Geometry: see drawing. Coordinates: mm, zero at the bounding-box minimum. A direction names the side the tool comes from. Give positions to 0.01 mm unless a question says otherwise; leave off trailing zeros. Loops run counter-clockwise (first coordinate to the right, second up) from the corner with the lowest first, then second, coordinate; pieces in that order, holes last. Notation, with made-up numbers: (89, 70.25) -> (132, 70.25) arc R31 cw to (132, 95.25) -> close; hole circle Ø10 at (-31.5, -4). An arc over 180 degrees is marked (long way). Answer in a Markdown table with one row per item. Add a question column.
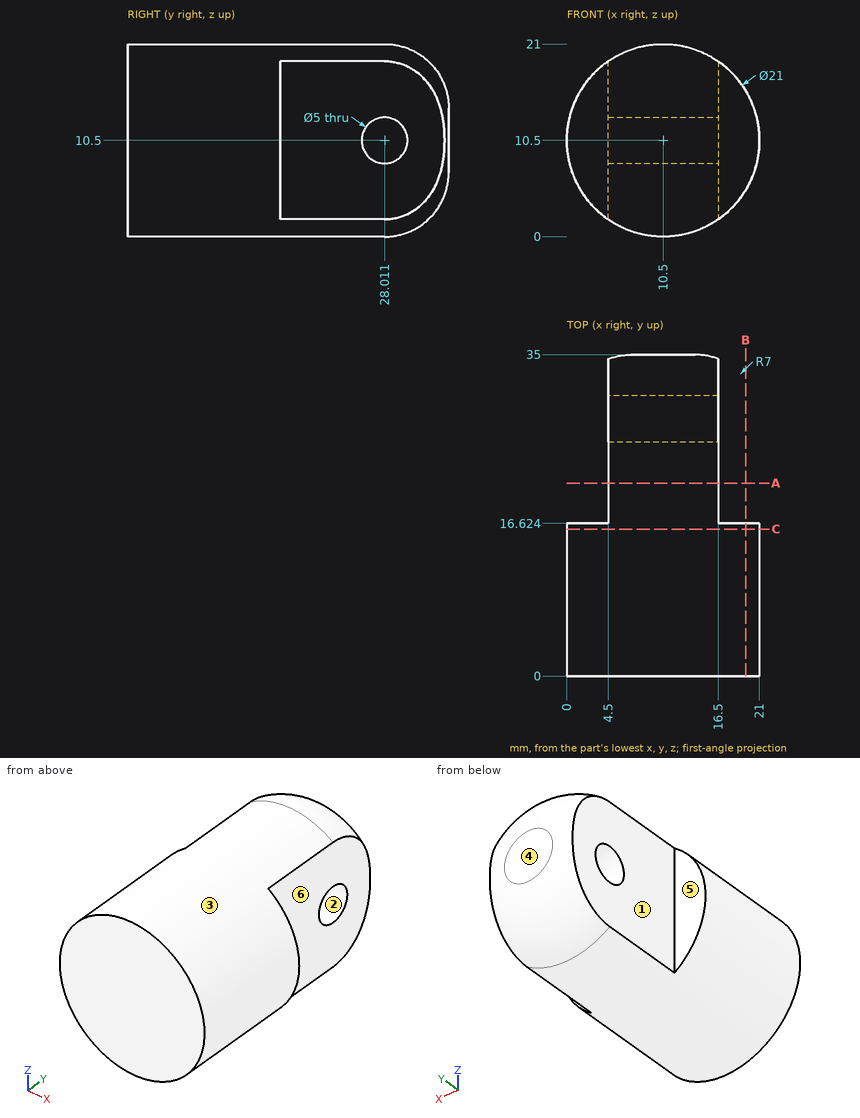
1) Pin query (flat end, axial travel): pin 1 (3.5 mm diameter, centred on x = 1.5, z = 10.5, fed in from +Y); pin 2 (5 mm diameter, centred on y = 22, z = 13.5, fed in from -X); pin 3 (3 mm diameter, centred on x = 16.5, y = 19.5, fed in from +Z). Return the tip coordinate at first contact, or that it passes through.
2) Pull-direction query (Z, two-part tool) for the marked faces 1, 2 and 3; classes: +Z half, -Z half, draft (parallel to the pull), parting line (faces both ways), or undercut.
3) Reachability of the marked faces 4, 5 and 6 from +Z, -Z, +X, -X, +Y, -Y: full face, straight path, thin tool, end or side. Return the list, or none.
4) Section C-C on y = 16. Output: boundary loops of the cut face in (x, z), and give its area (3 significant figures).
5) Section A-A on y = 21. Output: boundary loops of the cut face in (x, z).
6) Material intervals for line 1 along Y through (x, z) = (16.75, 5); line 2 along X through (y, z) = (27, 2.75); line 3 along Z through (x, y) = (14.75, 29) (1 decimal), sorted ascending.
7) Section B-B on x = 19.5. Output: boundary loops of the cut face in (y, z).
Working result:
| question | item | result |
|---|---|---|
| 1 | pin 1 | stops at y = 16.62 |
| 1 | pin 2 | stops at x = 4.5 |
| 1 | pin 3 | stops at z = 19.99 |
| 2 | face 1 | draft |
| 2 | face 2 | undercut |
| 2 | face 3 | parting line |
| 3 | face 4 | +Z, -Z, +X, -X, +Y |
| 3 | face 5 | +Z, -Z, -X, +Y |
| 3 | face 6 | +Z, -Z, +X, +Y |
| 4 | outline | circle Ø21 at (10.5, 10.5) |
| 4 | area | 346 mm2 |
| 5 | outline | (4.5, 1.88) arc R10.5 ccw to (16.5, 1.88) -> (16.5, 19.12) arc R10.5 ccw to (4.5, 19.12) -> close |
| 6 | line 1 | y = 0 to 16.62 |
| 6 | line 2 | x = 4.5 to 16.5 |
| 6 | line 3 | z = 1 to 8.2, 12.8 to 20 |
| 7 | outline | (0, 5.09) -> (16.62, 5.09) -> (16.62, 15.91) -> (0, 15.91) -> close |
